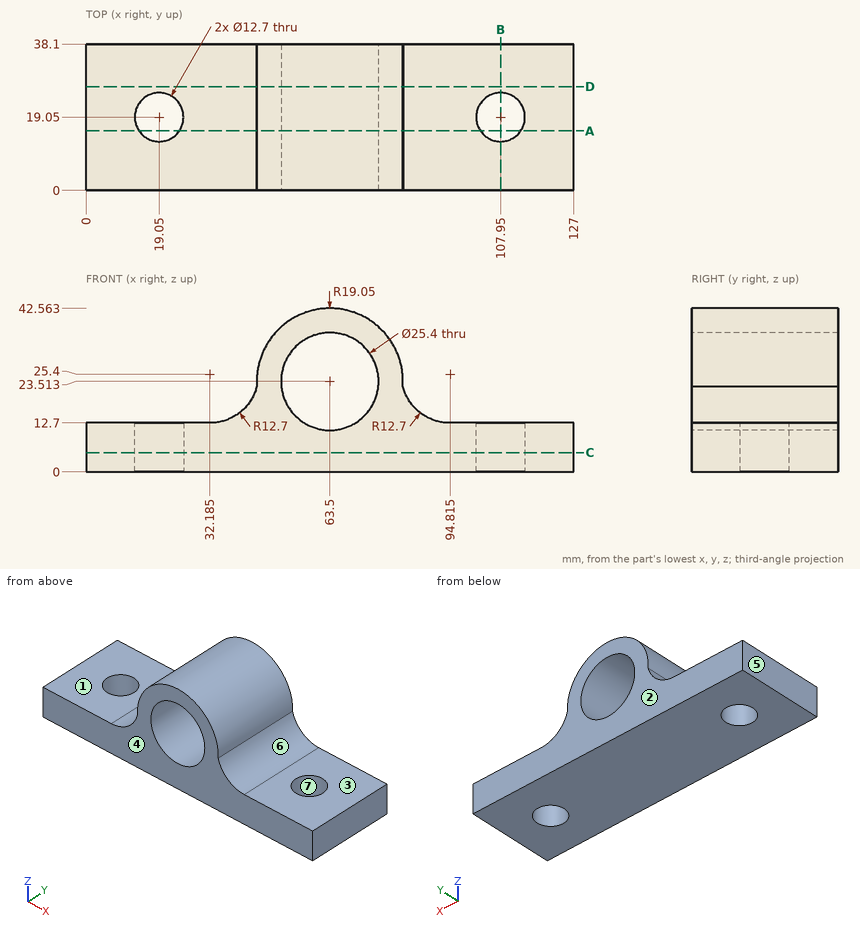
For this review, use the dimensioned drawing (mm, ordinates from the lowest corner) and the shaded views. A direction names the side the tool comes from. Coordinates: 2 decimals unless noted, no trailing zeros. Order: outer loops, then holes, each group sorted by start corner. A loop starts at its lowest first (then second) coordinate and runs counter-clockwise, first axis right, second up. Notation, with made-up numbers: (-5, -19.75) - (30, -19.75) arc R33 cw to (30, 8.25) - close; hole circle Ø2 at (3, 79). An arc over 180 degrees is marked (long way). Answer as a JSON object with one key per item and string values. Group by question number.
1. Clearance check with flat-ended pins moving along their axes: P1, Ø11.5, axis at x = 107.95, y = 19.05, coming from the +Z side (3 decimals); P2, Ø9.5, axis at x = 8, y = 25.5, coming from the +Z side; P3, Ø6, axis at x = 59.5, y = 30.5, coming from the -Z side; P4, Ø8, axis at y = 31.5, z = 25, coming from the -X side. State where each tip first meets the part, or that it passes through.
2. For the marked faces 1, 2 and 3, list the 3-axis set-ups (+Z, -Z, +X, -X, +Y, -Y) from which the entire face can be reached by the end or side of a thin tool; tool diameter is ignored.
3. For probe 1 along X at (y, z) = (19, 5); probe 2 along Y at (x, z) = (19.05, 6); probe 3 along Z at (x, y) = (97, 26.5), list the stretches that pass through material, from the lowest coordinate up.
4. The part is to be moulded in two halves that separate along X. For the marked faces 4, 5, 6 and 7, say which applies: pulls with the +X half, pulls with the -X half, needs draft (parallel to the pull), parting line crosses it, or undercut.
5. We need section A-A on y = 15.5. State the section outline as (x, z) points (3 decimals), then the cut area to 3 significant figures.
6. We need section B-B on x = 107.95. State the section outline as (y, z) points.
7. We need section C-C on z = 5. State the section outline as (x, y) points.
8. We need section D-D on y = 27. State the section outline as (x, z) points (3 decimals).
Final values:
{
 "1": {"P1": "through", "P2": "z = 12.7", "P3": "z = 0", "P4": "x = 44.1"},
 "2": {"face 1": "+Z, -X, +Y, -Y", "face 2": "+Z, -Z, +X, -X, +Y", "face 3": "+Z, +X, +Y, -Y"},
 "3": {"probe 1": "0 to 12.7, 25.4 to 101.6, 114.3 to 127", "probe 2": "0 to 12.7, 25.4 to 38.1", "probe 3": "0 to 12.7"},
 "4": {"face 4": "needs draft", "face 5": "pulls with the -X half", "face 6": "pulls with the +X half", "face 7": "undercut"},
 "5": {"outline": "(0, 0) - (13.785, 0) - (13.785, 12.7) - (0, 12.7) - close; (24.315, 0) - (102.685, 0) - (102.685, 12.7) - (94.815, 12.7) arc R12.7 cw to (82.509, 22.262) arc R19.05 ccw (long way) to (44.491, 22.262) arc R12.7 cw to (32.185, 12.7) - (24.315, 12.7) - close; (113.215, 0) - (127, 0) - (127, 12.7) - (113.215, 12.7) - close; hole circle Ø25.4 at (63.5, 23.513)", "area": "1,880 mm²"},
 "6": {"outline": "(0, 0) - (12.7, 0) - (12.7, 12.7) - (0, 12.7) - close; (25.4, 0) - (38.1, 0) - (38.1, 12.7) - (25.4, 12.7) - close"},
 "7": {"outline": "(0, 0) - (127, 0) - (127, 38.1) - (0, 38.1) - close; hole circle Ø12.7 at (19.05, 19.05); hole circle Ø12.7 at (107.95, 19.05)"},
 "8": {"outline": "(0, 0) - (127, 0) - (127, 12.7) - (94.815, 12.7) arc R12.7 cw to (82.509, 22.262) arc R19.05 ccw (long way) to (44.491, 22.262) arc R12.7 cw to (32.185, 12.7) - (0, 12.7) - close; hole circle Ø25.4 at (63.5, 23.513)"}
}
